Autodesk Inventor part; units mm, degrees
ref_plane "YZ Plane" through (0, 0, 0) normal (1, 0, 0) x (0, 1, 0)
ref_plane "XZ Plane" through (0, 0, 0) normal (0, 1, 0) x (-1, 0, 0)
ref_plane "XY Plane" through (0, 0, 0) normal (0, 0, 1) x (1, 0, 0)
sketch "Sketch1" plane through (0, 0, 0) normal (0, 0, 1) x (1, 0, 0)
  line L0 (519.5155, 1910) -> (-320.4845, 1910)
  line L1 (-320.4845, 1910) -> (-1085, 1150)
  line L2 (-1085, 0) -> (-1085, 1150)
  line L3 (1085, 0) -> (1085, 1372.7595)
  line L4 (519.5155, 1910) -> (1085, 1372.7595)
  line L5 (1085, 0) -> (-1085, 0)
  circle A0 centre (-865, 220) radius 200.5
  circle A1 centre (-493, 255) radius 38
  circle A2 centre (120, 955) radius 700 construction
  line L6 (499.31, 1277) -> (499.31, 1910) construction
  circle A3 centre (499.31, 1543.323) radius 30
  line L7 (1085, 955) -> (325, 955) construction
  circle A4 centre (120, 955) radius 205
  line L8 (120, 0) -> (120, 750) construction
  circle A5 centre (120, 955) radius 225 construction
  circle A6 centre (163.8953, 1175.6767) radius 6
  line L9 (120, 955) -> (120, 1180) construction
  line L10 (163.8953, 1175.6767) -> (120, 955) construction
  circle A7 centre (76.1047, 1175.6767) radius 6
  circle A8 centre (-5.0033, 1142.0807) radius 6
  circle A9 centre (-67.0807, 1080.0033) radius 6
  circle A10 centre (-100.6767, 998.8953) radius 6
  circle A11 centre (-100.6767, 911.1047) radius 6
  circle A12 centre (-67.0807, 829.9967) radius 6
  circle A13 centre (-5.0033, 767.9193) radius 6
  circle A14 centre (76.1047, 734.3233) radius 6
  circle A15 centre (163.8953, 734.3233) radius 6
  circle A16 centre (245.0033, 767.9193) radius 6
  circle A17 centre (307.0807, 829.9967) radius 6
  circle A18 centre (340.6767, 911.1047) radius 6
  circle A19 centre (340.6767, 998.8953) radius 6
  circle A20 centre (307.0807, 1080.0033) radius 6
  circle A21 centre (245.0033, 1142.0807) radius 6
  circle A22 centre (120, 955) radius 670 construction
  point P0 (0, 0)
  dimension "d69" = 1400
  dimension "d1" = 840
  dimension "d3" = 1150
  dimension "d14" = 76
  dimension "d15" = 1910
  dimension "d16" = 255
  dimension "d17" = 220
  dimension "d18" = 401
  dimension "d19" = 220
  dimension "d33" = 2170
  dimension "d49" = 372
  dimension "d51" = 780
  dimension "d52" = 1078
  dimension "d70" = 1584.31
  dimension "d71" = 60
  dimension "d74" = 760
  dimension "d75" = 410
  dimension "d76" = 750
  dimension "d77" = 450
  dimension "d78" = 12
  dimension "d79" = 11.25
  dimension "d82" = 360
  dimension "d84" = 465
extrude "Extrusion5" add sketch "Sketch1" along normal blind 10
equation "\"d17\" = d19"
properties part number "Left wall v2.0"
Model file for the job. Use its own axes, mm. Give positions to 0.01 mm unless a question says otherwise; leave off trailing zeros. Order: outer loops, then holes, each group sorted by start corner. A loop starts at its lowest first (then second) coordinate and runs counter-clockwise, first axis right, second up. Notation, with made-up numbers: (88.25, 52) - (93.25, 52) arc R22 cw to (93.25, 66) - close; hole circle Ø8 at (-14, -13.75). An arc over 180 degrees is marked (long way). Write item = value, one per line. Start each with the question number.
1. Cut at C-C, the plane y = 255. List the corners of the cut face in (x, z), and give its area (3 significant figures).
2. Cut at B-B, the plane x = 120. List the corners of the cut face in (y, z), and give its area (3 significant figures).
3. Cut at A-A, the plane y = 955. List the corners of the cut face in (x, z), and give its area (3 significant figures).
4. Two-plate mould, pull along X, no slides. Class faces 1 (the cylindrical face through (492.81, 1572.61, 4.93)), 2 (the flat face through (-15, 756, 10)), 3 (the flat face through (798.3, 1645.14, 4.93)), 4 (the cylindrical face through (-501.238, 292.096, 4.93)): pulls with the +X half, pulls with the -X half, needs draft (parallel to the pull), parting line crosses it, or undercut.
5. Cut at D-D, the plane z = 8.25. State how many separate pieces and enclosed holes the cut face has, and give its area (3 significant figures).
6. Probe line 1 along Y through (x, z) = (499.31, 5); line 2 along Y through (x, z) = (50, 1); line 3 along X through (y, z) = (132, 7.75). List the from-to ranges inside material, lowest first.
7. Drop a flat-ended pin along its axis: P1, Ø4, axis at x = 668.5, z = 4, coming from the +Y side. Give the stop position or say it passes through.
Taken from the geometry:
q1.outline = (-1085, 0) - (-1062.42, 0) - (-1062.42, 10) - (-1085, 10) - close; (-667.58, 0) - (-531, 0) - (-531, 10) - (-667.58, 10) - close; (-455, 0) - (1085, 0) - (1085, 10) - (-455, 10) - close
q1.area = 17,000 mm²
q2.outline = (0, 0) - (750, 0) - (750, 10) - (0, 10) - close; (1160, 0) - (1910, 0) - (1910, 10) - (1160, 10) - close
q2.area = 15,000 mm²
q3.outline = (-1085, 0) - (-85, 0) - (-85, 10) - (-1085, 10) - close; (325, 0) - (1085, 0) - (1085, 10) - (325, 10) - close
q3.area = 17,600 mm²
q4.face_1 = undercut
q4.face_2 = needs draft
q4.face_3 = pulls with the +X half
q4.face_4 = undercut
q5.separate_pieces = 1
q5.enclosed_holes = 20
q5.area = 3,430,000 mm²
q6.line_1 = 0 to 1513.32, 1573.32 to 1910
q6.line_2 = 0 to 762.32, 1147.68 to 1910
q6.line_3 = -1085 to -1045.16, -684.84 to 1085
q7.P1 = 1770.36
